Geometry check sheet. Reference: drawing and pictorial views, mm from the part's lowest x, y, z. Give positions to 0.01 mm unless a question says otherwise; leave off trailing zeros. Write each loop counter-clockwise with the first axis right and the second up, starting at its lowest first coordinate (ties: lowest second). Pieces come first, ordered by that corner, then holes.
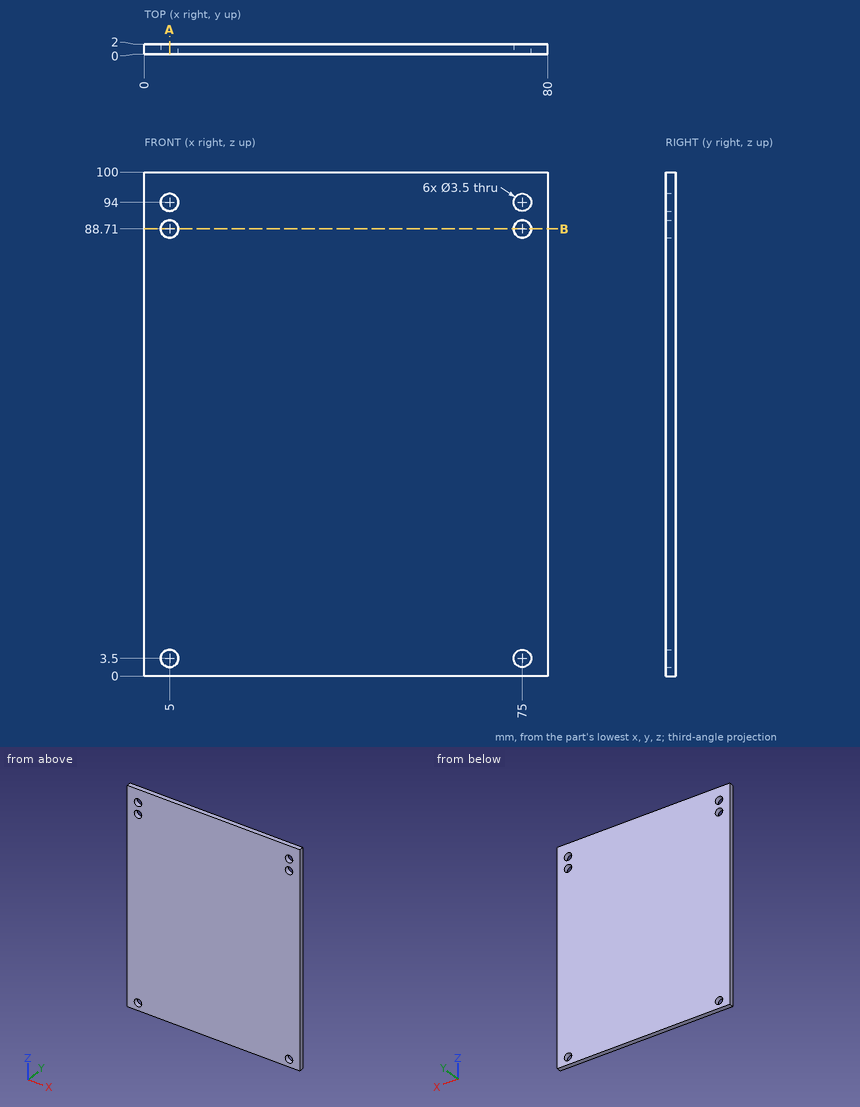
Item 1: Depth check by flat-ended pin: pin 1 (3 mm diameter, centred on x = 75, z = 88.71, fed in from -Y). Enter the tip coordinate at first touch or a pass-through.
Answer key:
pin 1: passes through
Item 2: Sectioned sample at B-B on z = 88.71. Record the cut outline in (x, y), then the cut area to 3 significant figures.
Answer key:
outline: (0, 0) - (3.25, 0) - (3.25, 2) - (0, 2) - close; (6.75, 0) - (73.25, 0) - (73.25, 2) - (6.75, 2) - close; (76.75, 0) - (80, 0) - (80, 2) - (76.75, 2) - close
area: 146 mm2
Item 3: Scan lines: line 1 along Z through (x, y) = (5, 1.55); line 2 along X through (y, z) = (0.6, 94); line 3 along Z through (x, y) = (6.5, 0.4). Record each from-to range of solid material in increasing order.
Answer key:
line 1: z = 0 to 1.75, 5.25 to 86.96, 90.46 to 92.25, 95.75 to 100
line 2: x = 0 to 3.25, 6.75 to 73.25, 76.75 to 80
line 3: z = 0 to 2.6, 4.4 to 87.81, 89.61 to 93.1, 94.9 to 100
Item 4: Sectioned sample at A-A on x = 5. Record the cut outline in (y, z).
Answer key:
outline: (0, 0) - (2, 0) - (2, 1.75) - (0, 1.75) - close; (0, 5.25) - (2, 5.25) - (2, 86.96) - (0, 86.96) - close; (0, 90.46) - (2, 90.46) - (2, 92.25) - (0, 92.25) - close; (0, 95.75) - (2, 95.75) - (2, 100) - (0, 100) - close
